The model under review builds one solid part; all positions refer to its coordinate system, in mm. A direction names the side the tool comes from. Coordinates: 2 decimals unless noted, no trailing zeros. Order: outer loops, then holes, each group sorted by start corner. A loop starts at its lowest first (then second) coordinate and runs counter-clockwise, first axis right, second up. Notation, with made-up numbers: (-19, 29.5) -> (18, 29.5) arc R14 cw to (18, 56.5) -> close; hole circle Ø5 at (-25, 19.5). An arc over 180 degrees is marked (long way). Use one line per item in the form item = value. Start each with the question number.
(1) Mouldability with a two-part tool opening along Z and no side actions: class faces 1 (the cylindrical face through (-2.73, -32.18, 21.94)), 2 (the flat face through (0.1, -31.8, 26)), 3 (the flat face through (-181.5, 57.8, 125.4)) as +Z half, -Z half, draft (parallel to the pull), parting line (faces both ways), or undercut.
(2) Take a section at C-C (z = 90). State the section outline as (x, y) points.
(3) Take a section at A-A (x = -89.5). State the section outline as (y, z) points.
(4) For faces 4 (the flat face through (-3, 158, 89)), 5 (the flat face through (-3, -158, 89)), 6 (the flat face through (-153, -2, 184)), 7 (the flat face through (-173, -145, 157)), 8 (the flat face through (-2, -125, 180)), list the 3-axis set-ups (+Z, -Z, +X, -X, +Y, -Y) from which the entire face can be reached by the end or side of a thin tool; tool diameter is ignored.
(5) Insertion check: pin 1 Ø6 at (x, y) = (-173.31, 144.5) entering from +Z; pin 2 Ø10 at (x, y) = (25, -11) entering from +Z. Each pin has a flat end and moves straight along its axis. Give the tip position at first contact, or say it passes through.
(6) Take a section at B-B (y = -104). State the section outline as (x, z) points.
(7) Wall thickness on line 1 along Y through (x, z) = (181, 145); line 2 along Y through (x, z) = (-158, 91); line 3 along X through (y, z) = (86, 23.5): over which ranges is each line inside the solid? List them lowest first.
(8) Take a section at D-D (x = 84). State the section outline as (y, z) points.
```python
from build123d import *

# Parameters (mm, degrees)
CROQUIS1_W                     = 379
CROQUIS1_H                     = 316
SALIENTE_EXTRUIR1_DEPTH        = 180
VACIADO1_T                     = -8
CROQUIS2_R                     = 35
CORTAR_EXTRUIR4_DEPTH          = 20
CROQUIS4_R                     = 45
CROQUIS4_R_2                   = 40
SALIENTE_EXTRUIR4_DEPTH        = 10
CORTAR_EXTRUIR6_START          = -10
CROQUIS6_R                     = 45
CORTAR_EXTRUIR6_DEPTH          = 10
CROQUIS7_R                     = 24
CROQUIS7_R_2                   = 21
SALIENTE_EXTRUIR9_DEPTH        = 18
CROQUIS11_W                    = 363
CROQUIS11_H                    = 300
CROQUIS11_W_2                  = 300
CROQUIS11_H_2                  = 250
SALIENTE_EXTRUIR10_DEPTH       = 8
CROQUIS12_W                    = 306
CROQUIS12_H                    = 256
CROQUIS12_W_2                  = 300
CROQUIS12_H_2                  = 250
SALIENTE_EXTRUIR11_DEPTH       = 8
CROQUIS20_R                    = 21
CROQUIS20_R_2                  = 18.5
SALIENTE_EXTRUIR19_DEPTH       = 10
CROQUIS32_R                    = 5
SALIENTE_EXTRUIR22_DEPTH       = 10
TALADRO_ROSCADO_M63_AT_2_COUNT = 2
TALADRO_ROSCADO_M63_AT_2_PITCH = 110
TALADRO_ROSCADO_M63_AT_3_COUNT = 2
TALADRO_ROSCADO_M63_AT_3_PITCH = 159.138304628
TALADRO_ROSCADO_M63_AT_4_COUNT = 2
TALADRO_ROSCADO_M63_AT_4_PITCH = 115
CROQUIS28_W                    = 125
CROQUIS28_H                    = 225
CORTAR_EXTRUIR7_DEPTH          = 8
CROQUIS29_W                    = 10
CROQUIS29_H                    = 20
CORTAR_EXTRUIR9_DEPTH          = 8
CROQUIS30_R                    = 2
SALIENTE_EXTRUIR20_DEPTH       = 9
CROQUIS31_R                    = 2
SALIENTE_EXTRUIR21_DEPTH       = 9
SALIENTE_EXTRUIR23_START       = -8
CROQUIS33_R                    = 5
SALIENTE_EXTRUIR23_DEPTH       = 15
TALADRO_ROSCADO_M64_D          = 5
TALADRO_ROSCADO_M64_DEPTH      = 17
TALADRO_ROSCADO_M64_TIP        = 1.502151548


with BuildPart() as part:
    # Croquis1 → Saliente-Extruir1 (new body)
    with BuildSketch(Plane.XY):
        Rectangle(CROQUIS1_W, CROQUIS1_H)
    extrude(amount=SALIENTE_EXTRUIR1_DEPTH)

    # Vaciado1
    vaciado1_openings = [part.faces().sort_by_distance(p)[0] for p in [
        (0, 0, 180),
    ]]
    offset(amount=VACIADO1_T, openings=vaciado1_openings, kind=Kind.INTERSECTION)

    # Croquis2 → Cortar-Extruir4 (cut)
    with BuildSketch(Plane.ZY.offset(189.5)):
        with Locations((90, 58)):
            Circle(CROQUIS2_R)
    extrude(amount=-CORTAR_EXTRUIR4_DEPTH, mode=Mode.SUBTRACT)

    # Croquis4 → Saliente-Extruir4 (add)
    with BuildSketch(Plane(origin=(-181.5, 0, 0), x_dir=(0, 0, -1), z_dir=(1, 0, 0))):
        with Locations((-90, 58)):
            Circle(CROQUIS4_R)
        with Locations((-90, 58)):
            Circle(CROQUIS4_R_2, mode=Mode.SUBTRACT)
    extrude(amount=SALIENTE_EXTRUIR4_DEPTH)

    # Croquis6 → Cortar-Extruir6 (cut)
    with BuildSketch(Plane(origin=(189.5, 0, 0), x_dir=(0, 0, -1), z_dir=(1, 0, 0)).offset(CORTAR_EXTRUIR6_START)):
        with Locations((-90, 58)):
            Circle(CROQUIS6_R)
    extrude(amount=CORTAR_EXTRUIR6_DEPTH, mode=Mode.SUBTRACT)

    # Croquis7 → Saliente-Extruir9 (add)
    with BuildSketch(Plane.XY.offset(8)):
        with Locations(Location((0, -53, 0), (0, 0, 180))):
            Circle(CROQUIS7_R)
        with Locations((0, -53)):
            Circle(CROQUIS7_R_2, mode=Mode.SUBTRACT)
    extrude(amount=SALIENTE_EXTRUIR9_DEPTH)

    # Croquis11 → Saliente-Extruir10 (add)
    with BuildSketch(Plane.XY.offset(180)):
        Rectangle(CROQUIS11_W, CROQUIS11_H)
        Rectangle(CROQUIS11_W_2, CROQUIS11_H_2, mode=Mode.SUBTRACT)
    extrude(amount=-SALIENTE_EXTRUIR10_DEPTH)

    # Croquis12 → Saliente-Extruir11 (add)
    with BuildSketch(Plane.XY.offset(180)):
        Rectangle(CROQUIS12_W, CROQUIS12_H)
        Rectangle(CROQUIS12_W_2, CROQUIS12_H_2, mode=Mode.SUBTRACT)
    extrude(amount=SALIENTE_EXTRUIR11_DEPTH)

    # Croquis20 → Saliente-Extruir19 (add)
    with BuildSketch(Plane.XY.offset(8)):
        with Locations((0, -53)):
            Circle(CROQUIS20_R)
        with Locations((0, -53)):
            Circle(CROQUIS20_R_2, mode=Mode.SUBTRACT)
    extrude(amount=SALIENTE_EXTRUIR19_DEPTH)

    # Croquis32 → Saliente-Extruir22 (add)
    with BuildSketch(Plane(origin=(-181.5, 0, 0), x_dir=(0, 0, -1), z_dir=(1, 0, 0))):
        with Locations((-35, 115.5)):
            Circle(CROQUIS32_R)
        with Locations((-145, 115.5)):
            Circle(CROQUIS32_R)
        with Locations((-145, 0.5)):
            Circle(CROQUIS32_R)
        with Locations((-35, 0.5)):
            Circle(CROQUIS32_R)
    saliente_extruir22 = extrude(amount=SALIENTE_EXTRUIR22_DEPTH)

    # Croquis26 → Taladro roscado M63 (revolve, cut)
    with BuildSketch(Plane(origin=(-189.5, 115.5, 35), x_dir=(0, 0, 1), z_dir=(0, 1, 0))):
        Polygon((0, 0), (0, 15.502151548), (2.5, 14), (2.5, 0), align=None)
    taladro_roscado_m63 = revolve(axis=Axis((-195.85, 115.5, 35), (1, 0, 0)), mode=Mode.SUBTRACT)

    # Taladro roscado M63 at 2: Taladro roscado M63 ×2
    with Locations(*[(0, 0, i * TALADRO_ROSCADO_M63_AT_2_PITCH) for i in range(1, TALADRO_ROSCADO_M63_AT_2_COUNT)]):
        add(taladro_roscado_m63, mode=Mode.SUBTRACT)

    # Taladro roscado M63 at 3: Taladro roscado M63 ×2
    with Locations(*[Vector(0, -0.7226418571476992, 0.6912226459673645) * (i * TALADRO_ROSCADO_M63_AT_3_PITCH) for i in range(1, TALADRO_ROSCADO_M63_AT_3_COUNT)]):
        add(taladro_roscado_m63, mode=Mode.SUBTRACT)

    # Taladro roscado M63 at 4: Taladro roscado M63 ×2
    with Locations(*[(0, -i * TALADRO_ROSCADO_M63_AT_4_PITCH, 0) for i in range(1, TALADRO_ROSCADO_M63_AT_4_COUNT)]):
        add(taladro_roscado_m63, mode=Mode.SUBTRACT)

    # Croquis28 → Cortar-Extruir7 (cut)
    with BuildSketch(Plane(origin=(0, 0, 0), x_dir=(-1, 0, 0), z_dir=(0, 0, -1))):
        with Locations((106, 0)):
            Rectangle(CROQUIS28_W, CROQUIS28_H)
    extrude(amount=-CORTAR_EXTRUIR7_DEPTH, mode=Mode.SUBTRACT)

    # Croquis29 → Cortar-Extruir9 (cut)
    with BuildSketch(Plane(origin=(0, 0, 0), x_dir=(-1, 0, 0), z_dir=(0, 0, -1))):
        with Locations((173.5, 52.5)):
            Rectangle(CROQUIS29_W, CROQUIS29_H)
        with Locations((173.5, -52.5)):
            Rectangle(CROQUIS29_W, CROQUIS29_H)
    extrude(amount=-CORTAR_EXTRUIR9_DEPTH, mode=Mode.SUBTRACT)

    # Croquis30 → Saliente-Extruir20 (add)
    with BuildSketch(Plane(origin=(0, 42.5, 0), x_dir=(1, 0, 0), z_dir=(0, 1, 0))):
        with Locations(Location((-174.5, -4, 0), (0, 0, 90))):
            Circle(CROQUIS30_R)
    extrude(amount=SALIENTE_EXTRUIR20_DEPTH)

    # Croquis31 → Saliente-Extruir21 (add)
    with BuildSketch(Plane(origin=(0, -62.5, 0), x_dir=(1, 0, 0), z_dir=(0, 1, 0))):
        with Locations(Location((-174.5, -4, 0), (0, 0, 90))):
            Circle(CROQUIS31_R)
    extrude(amount=SALIENTE_EXTRUIR21_DEPTH)

    # Simetría1: Saliente-Extruir22 across plane
    add(saliente_extruir22.mirror(Plane(origin=(0, 0, 0), x_dir=(0, 0, 1), z_dir=(1, 0, 0))))

    # Croquis33 → Saliente-Extruir23 (add)
    with BuildSketch(Plane.XY.offset(180).offset(SALIENTE_EXTRUIR23_START)):
        with Locations(Location((0, 144.5, 0), (0, 0, 180))):
            Circle(CROQUIS33_R)
        with Locations(Location((0, -144.5, 0), (0, 0, 180))):
            Circle(CROQUIS33_R)
        with Locations(Location((173.308544304, -144.5, 0), (0, 0, 180))):
            Circle(CROQUIS33_R)
        with Locations(Location((173.308544304, 144.5, 0), (0, 0, 180))):
            Circle(CROQUIS33_R)
        with Locations(Location((-173.308544304, 144.5, 0), (0, 0, 180))):
            Circle(CROQUIS33_R)
        with Locations(Location((-173.308544304, -144.5, 0), (0, 0, 180))):
            Circle(CROQUIS33_R)
    extrude(amount=-SALIENTE_EXTRUIR23_DEPTH)

    # Taladro roscado M64
    with Locations(Plane(origin=(-173.308544304, 144.5, 180), x_dir=(1, 0, 0), z_dir=(0, 0, 1))):
        with Locations((0, 0), (173.308544304, 0), (346.617088608, 0), (346.617088608, -289), (173.308544304, -289), (0, -289)):
            Hole(TALADRO_ROSCADO_M64_D / 2, depth=TALADRO_ROSCADO_M64_DEPTH)
            with Locations((0, 0, -(TALADRO_ROSCADO_M64_DEPTH + TALADRO_ROSCADO_M64_TIP / 2))):  # 118° drill point
                Cone(0, TALADRO_ROSCADO_M64_D / 2, TALADRO_ROSCADO_M64_TIP, mode=Mode.SUBTRACT)

    # Simetría2: Taladro roscado M63 across plane
    add(taladro_roscado_m63.mirror(Plane(origin=(0, 0, 0), x_dir=(0, 0, 1), z_dir=(1, 0, 0))), mode=Mode.SUBTRACT)

    # Simetría2 copy 1 sketch → Simetría2 copy 1 (revolve, cut)
    with BuildSketch(Plane(origin=(189.5, 115.5, 145), x_dir=(0, 0, 1), z_dir=(0, 1, 0))):
        Polygon((0, 0), (0, -15.502151548), (2.5, -14), (2.5, 0), align=None)
    revolve(axis=Axis((195.85, 115.5, 145), (1, 0, 0)), mode=Mode.SUBTRACT)

    # Simetría2 copy 2 sketch → Simetría2 copy 2 (revolve, cut)
    with BuildSketch(Plane(origin=(189.5, 0.5, 145), x_dir=(0, 0, 1), z_dir=(0, 1, 0))):
        Polygon((0, 0), (0, -15.502151548), (2.5, -14), (2.5, 0), align=None)
    revolve(axis=Axis((195.85, 0.5, 145), (1, 0, 0)), mode=Mode.SUBTRACT)

    # Simetría2 copy 3 sketch → Simetría2 copy 3 (revolve, cut)
    with BuildSketch(Plane(origin=(189.5, 0.5, 35), x_dir=(0, 0, 1), z_dir=(0, 1, 0))):
        Polygon((0, 0), (0, -15.502151548), (2.5, -14), (2.5, 0), align=None)
    revolve(axis=Axis((195.85, 0.5, 35), (1, 0, 0)), mode=Mode.SUBTRACT)


solid = part.part
```
Findings:
q1.face_1 = draft
q1.face_2 = +Z half
q1.face_3 = undercut
q2.outline = (-189.5, -158) -> (189.5, -158) -> (189.5, 13) -> (181.5, 13) -> (181.5, -150) -> (-181.5, -150) -> (-181.5, 13) -> (-171.5, 13) -> (-171.5, 18) -> (-181.5, 18) -> (-181.5, 23) -> (-189.5, 23) -> close; (-189.5, 93) -> (-181.5, 93) -> (-181.5, 98) -> (-171.5, 98) -> (-171.5, 103) -> (-181.5, 103) -> (-181.5, 150) -> (181.5, 150) -> (181.5, 103) -> (189.5, 103) -> (189.5, 158) -> (-189.5, 158) -> close
q3.outline = (-158, 0) -> (-112.5, 0) -> (-112.5, 8) -> (-150, 8) -> (-150, 172) -> (-125, 172) -> (-125, 188) -> (-128, 188) -> (-128, 180) -> (-158, 180) -> close; (112.5, 0) -> (158, 0) -> (158, 180) -> (128, 180) -> (128, 188) -> (125, 188) -> (125, 172) -> (150, 172) -> (150, 8) -> (112.5, 8) -> close
q4.face_4 = +Z, -Z, +X, -X, +Y
q4.face_5 = +Z, -Z, +X, -X, -Y
q4.face_6 = +Z, -X, +Y, -Y
q4.face_7 = none
q4.face_8 = +Z
q5.pin_1 = 180
q5.pin_2 = 8
q6.outline = (-189.5, 0) -> (-168.5, 0) -> (-168.5, 8) -> (-181.5, 8) -> (-181.5, 172) -> (-150, 172) -> (-150, 188) -> (-153, 188) -> (-153, 180) -> (-189.5, 180) -> close; (-43.5, 0) -> (189.5, 0) -> (189.5, 180) -> (153, 180) -> (153, 188) -> (150, 188) -> (150, 172) -> (181.5, 172) -> (181.5, 8) -> (-43.5, 8) -> close
q7.line_1 = -158 to -150, -4.5 to -2, 3 to 5.5, 110.5 to 113, 118 to 120.5, 150 to 158
q7.line_2 = -158 to -150, 150 to 158
q7.line_3 = -189.5 to -181.5, 181.5 to 189.5
q8.outline = (-158, 0) -> (158, 0) -> (158, 180) -> (128, 180) -> (128, 188) -> (125, 188) -> (125, 172) -> (150, 172) -> (150, 8) -> (-150, 8) -> (-150, 172) -> (-125, 172) -> (-125, 188) -> (-128, 188) -> (-128, 180) -> (-158, 180) -> close
